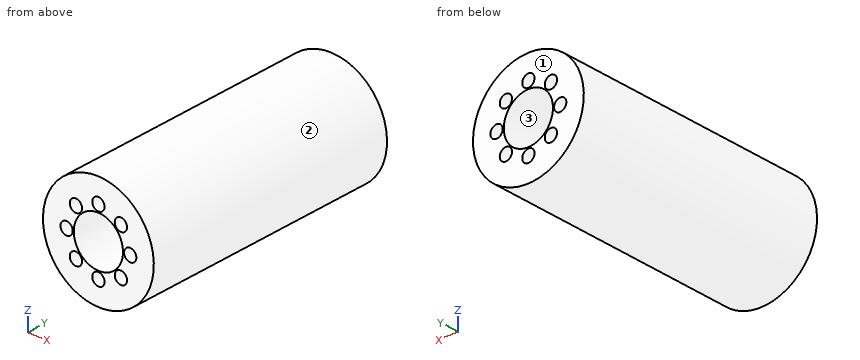
```python
from build123d import *

# Parameters (mm, degrees)
SKETCH_1_R          = 67.58
SKETCH_1_R_2        = 30
EXTRUDE_1_DEPTH     = 319
CUT_EXTRUDE_1_REACH = 335.009
SKETCH_2_R          = 7.5


with BuildPart() as part:
    # 草图1 → 凸台-拉伸1 (new body)
    with BuildSketch(Plane(origin=(0, 0, 0), x_dir=(1, 0, 0), z_dir=(0, 1, 0))):
        with Locations(Location((0, 0, 0), (0, 0, 270))):
            Circle(SKETCH_1_R)
        with Locations(Location((0, 0, 0), (0, 0, 270))):
            Circle(SKETCH_1_R_2, mode=Mode.SUBTRACT)
    extrude(amount=EXTRUDE_1_DEPTH)

    # 草图2 → 切除-拉伸1 (cut, up to next)
    with BuildSketch(Plane(origin=(0, 319, 0), x_dir=(1, 0, 0), z_dir=(0, 1, 0)), mode=Mode.PRIVATE) as cut_extrude_1_sk1:
        with Locations(Location((-38.8, 0, 0), (0, 0, 270))):
            Circle(SKETCH_2_R)
    cut_extrude_1_tool1 = extrude(cut_extrude_1_sk1.sketch, amount=-CUT_EXTRUDE_1_REACH, mode=Mode.PRIVATE) & part.part
    # 草图2 → 切除-拉伸1 (cut, up to next)
    with BuildSketch(Plane(origin=(0, 319, 0), x_dir=(1, 0, 0), z_dir=(0, 1, 0)), mode=Mode.PRIVATE) as cut_extrude_1_sk2:
        with Locations(Location((-27.43574311, 27.43574311, 0), (0, 0, 270))):
            Circle(SKETCH_2_R)
    cut_extrude_1_tool2 = extrude(cut_extrude_1_sk2.sketch, amount=-CUT_EXTRUDE_1_REACH, mode=Mode.PRIVATE) & part.part
    # 草图2 → 切除-拉伸1 (cut, up to next)
    with BuildSketch(Plane(origin=(0, 319, 0), x_dir=(1, 0, 0), z_dir=(0, 1, 0)), mode=Mode.PRIVATE) as cut_extrude_1_sk3:
        with Locations(Location((0, 38.8, 0), (0, 0, 270))):
            Circle(SKETCH_2_R)
    cut_extrude_1_tool3 = extrude(cut_extrude_1_sk3.sketch, amount=-CUT_EXTRUDE_1_REACH, mode=Mode.PRIVATE) & part.part
    # 草图2 → 切除-拉伸1 (cut, up to next)
    with BuildSketch(Plane(origin=(0, 319, 0), x_dir=(1, 0, 0), z_dir=(0, 1, 0)), mode=Mode.PRIVATE) as cut_extrude_1_sk4:
        with Locations(Location((27.43574311, 27.43574311, 0), (0, 0, 270))):
            Circle(SKETCH_2_R)
    cut_extrude_1_tool4 = extrude(cut_extrude_1_sk4.sketch, amount=-CUT_EXTRUDE_1_REACH, mode=Mode.PRIVATE) & part.part
    # 草图2 → 切除-拉伸1 (cut, up to next)
    with BuildSketch(Plane(origin=(0, 319, 0), x_dir=(1, 0, 0), z_dir=(0, 1, 0)), mode=Mode.PRIVATE) as cut_extrude_1_sk5:
        with Locations(Location((38.8, 0, 0), (0, 0, 270))):
            Circle(SKETCH_2_R)
    cut_extrude_1_tool5 = extrude(cut_extrude_1_sk5.sketch, amount=-CUT_EXTRUDE_1_REACH, mode=Mode.PRIVATE) & part.part
    # 草图2 → 切除-拉伸1 (cut, up to next)
    with BuildSketch(Plane(origin=(0, 319, 0), x_dir=(1, 0, 0), z_dir=(0, 1, 0)), mode=Mode.PRIVATE) as cut_extrude_1_sk6:
        with Locations(Location((27.43574311, -27.43574311, 0), (0, 0, 270))):
            Circle(SKETCH_2_R)
    cut_extrude_1_tool6 = extrude(cut_extrude_1_sk6.sketch, amount=-CUT_EXTRUDE_1_REACH, mode=Mode.PRIVATE) & part.part
    # 草图2 → 切除-拉伸1 (cut, up to next)
    with BuildSketch(Plane(origin=(0, 319, 0), x_dir=(1, 0, 0), z_dir=(0, 1, 0)), mode=Mode.PRIVATE) as cut_extrude_1_sk7:
        with Locations(Location((0, -38.8, 0), (0, 0, 270))):
            Circle(SKETCH_2_R)
    cut_extrude_1_tool7 = extrude(cut_extrude_1_sk7.sketch, amount=-CUT_EXTRUDE_1_REACH, mode=Mode.PRIVATE) & part.part
    # 草图2 → 切除-拉伸1 (cut, up to next)
    with BuildSketch(Plane(origin=(0, 319, 0), x_dir=(1, 0, 0), z_dir=(0, 1, 0)), mode=Mode.PRIVATE) as cut_extrude_1_sk8:
        with Locations(Location((-27.43574311, -27.43574311, 0), (0, 0, 270))):
            Circle(SKETCH_2_R)
    cut_extrude_1_tool8 = extrude(cut_extrude_1_sk8.sketch, amount=-CUT_EXTRUDE_1_REACH, mode=Mode.PRIVATE) & part.part
    add(cut_extrude_1_tool1.solids().sort_by_distance((-38.8, 319, 0))[0], mode=Mode.SUBTRACT)
    add(cut_extrude_1_tool2.solids().sort_by_distance((-27.435743, 319, -27.435743))[0], mode=Mode.SUBTRACT)
    add(cut_extrude_1_tool3.solids().sort_by_distance((0, 319, -38.8))[0], mode=Mode.SUBTRACT)
    add(cut_extrude_1_tool4.solids().sort_by_distance((27.435743, 319, -27.435743))[0], mode=Mode.SUBTRACT)
    add(cut_extrude_1_tool5.solids().sort_by_distance((38.8, 319, 0))[0], mode=Mode.SUBTRACT)
    add(cut_extrude_1_tool6.solids().sort_by_distance((27.435743, 319, 27.435743))[0], mode=Mode.SUBTRACT)
    add(cut_extrude_1_tool7.solids().sort_by_distance((0, 319, 38.8))[0], mode=Mode.SUBTRACT)
    add(cut_extrude_1_tool8.solids().sort_by_distance((-27.435743, 319, 27.435743))[0], mode=Mode.SUBTRACT)


solid = part.part
```
The model under review builds one solid part; all positions refer to its coordinate system, in mm. Face numbers are marked on the shaded views. Round coordinates to 2 decimals unless told otherwise and drop trailing zeros. Write each loop counter-clockwise with the first axis right and the second up, starting at its lowest first coordinate (ties: lowest second). Pieces come first, ordered by that corner, then holes.
(1) Wall thickness on L1, parallel to X at y = 234, z = 0; L2, parallel to X at y = 206.5, z = -22.5; L3, parallel to Z at x = -24.5, y = 278: over which ranges is each line inside the solid? List them lowest first.
(2) We need section B-B on z = -13.5. Give the boundary of the cut face in (x, y).
(3) We need section D-D on x = 38.8. Give the boundary of the cut face in (y, z).
(4) We need section A-A on x = 0. Give the boundary of the cut face in (y, z).
(5) Insertion check: pin 1 (4 mm diameter, centred on x = -18.5, y = 283, fed in from -Z); pin 2 (2 mm diameter, centred on y = 70.5, z = 2.5, fed in from +X); pin 3 (8 mm diameter, centred on y = 248.5, z = 49.5, fed in from +X); pin 4 (12 mm diameter, centred on x = 27.44, z = -27.44, fed in from -Y). Each pin has a flat end and moves straight along its axis. Give the tip position at first contact, or say it passes through.
(6) Mouldability with a two-part tool opening along X and no side actions: class the marked faces 1, 2 and 3 as +X half, -X half, draft (parallel to the pull), parting line (faces both ways), or undercut.
(7) We need section C-C on y = 216. Give the number of separate pieces and of enclosed holes in the cut face, and give its area (3 significant figures).
Findings below:
1. L1: x = -67.58 to -46.3, -31.3 to -30, 30 to 31.3, 46.3 to 67.58
1. L2: x = -63.72 to -33.08, -21.79 to -19.84, 19.84 to 21.79, 33.08 to 63.72
1. L3: z = -62.98 to -34.34, -20.53 to -17.31, 17.31 to 20.53, 34.34 to 62.98
2. outline: (-66.22, 0) - (-26.79, 0) - (-26.79, 319) - (-66.22, 319) - close; (26.79, 0) - (66.22, 0) - (66.22, 319) - (26.79, 319) - close
3. outline: (0, -55.33) - (319, -55.33) - (319, -7.5) - (0, -7.5) - close; (0, 7.5) - (319, 7.5) - (319, 55.33) - (0, 55.33) - close
4. outline: (0, -67.58) - (319, -67.58) - (319, -46.3) - (0, -46.3) - close; (0, -31.3) - (319, -31.3) - (319, -30) - (0, -30) - close; (0, 30) - (319, 30) - (319, 31.3) - (0, 31.3) - close; (0, 46.3) - (319, 46.3) - (319, 67.58) - (0, 67.58) - close
5. pin 1: stops at z = -65.53
5. pin 2: stops at x = 67.56
5. pin 3: stops at x = 49.97
5. pin 4: passes through
6. face 1: draft
6. face 2: parting line
6. face 3: undercut
7. separate pieces: 1
7. enclosed holes: 9
7. area: 10,100 mm2
